from build123d import *

# Parameters (mm, degrees)
BOSS_EXTRUDE2_DEPTH = 50.25
CUT_EXTRUDE3_DEPTH  = 37
SKETCH6_W           = 6.4
SKETCH6_H           = 6.4
SKETCH6_R           = 1.7
BOSS_EXTRUDE3_DEPTH = 3
SKETCH8_W           = 102.5
SKETCH8_H           = 6.25
BOSS_EXTRUDE4_DEPTH = 2
SKETCH7_R           = 2
CUT_EXTRUDE4_DEPTH  = 7


with BuildPart() as part:
    # Sketch4 → Boss-Extrude2 (new body)
    with BuildSketch(Plane.XY):
        Polygon((3.25, 0), (105.75, 0), (105.75, 6.25), (103.25, 6.25), (103.25, 8.75), (109, 8.75), (109, 40), (0, 40), (0, 8.75), (5.75, 8.75), (5.75, 6.25), (3.25, 6.25), align=None)
    extrude(amount=BOSS_EXTRUDE2_DEPTH)

    # Sketch5 → Cut-Extrude3 (cut)
    with BuildSketch(Plane.XZ):
        Polygon((3.25, 0), (8.418575633, 0), (100.815935432, 0), (105.75, 0), (105.75, 45.25), (100.75, 45.25), (100.75, 47.25), (8.25, 47.25), (8.25, 45.25), (3.25, 45.25), align=None)
    extrude(amount=-CUT_EXTRUDE3_DEPTH, mode=Mode.SUBTRACT)

    # Sketch6 → Boss-Extrude3 (add)
    # profile 1 of 2: a face of its own
    with BuildSketch(Plane(origin=(0, 0, 0), x_dir=(-1, 0, 0), z_dir=(0, 0, -1))):
        with Locations((-105.8, 43.2)):
            Rectangle(SKETCH6_W, SKETCH6_H)
        with Locations((-105.8, 43.2)):
            Circle(SKETCH6_R, mode=Mode.SUBTRACT)
    # profile 2 of 2: a face of its own
    with BuildSketch(Plane(origin=(0, 0, 0), x_dir=(-1, 0, 0), z_dir=(0, 0, -1))):
        with Locations((-3.2, 43.2)):
            Rectangle(SKETCH6_W, SKETCH6_H)
        with Locations((-3.2, 43.2)):
            Circle(SKETCH6_R, mode=Mode.SUBTRACT)
    extrude(amount=-BOSS_EXTRUDE3_DEPTH)

    # Sketch8 → Boss-Extrude4 (add)
    with BuildSketch(Plane.XY.offset(50.25)):
        with Locations((54.5, 3.125)):
            Rectangle(SKETCH8_W, SKETCH8_H)
    extrude(amount=BOSS_EXTRUDE4_DEPTH)

    # Sketch7 → Cut-Extrude4 (cut)
    with BuildSketch(Plane(origin=(105.75, 0, 0), x_dir=(0, 0, -1), z_dir=(1, 0, 0))):
        with Locations((-48.75, 3.125)):
            Circle(SKETCH7_R)
    cut_extrude4 = extrude(amount=-CUT_EXTRUDE4_DEPTH, mode=Mode.SUBTRACT)

    # Mirror1: Cut-Extrude4 across plane
    add(cut_extrude4.mirror(Plane(origin=(54.5, 0, 0), x_dir=(0, 0, 1), z_dir=(1, 0, 0))), mode=Mode.SUBTRACT)


solid = part.part
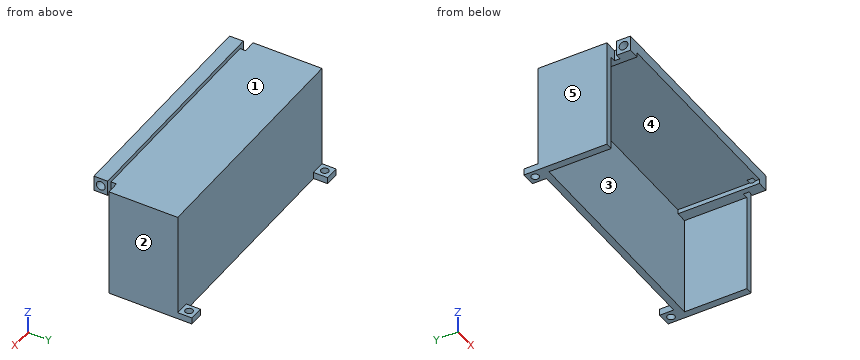
Source: CAD feature listing. Evaluate the final solid. Frame: model axes, mm. Face numbers are marked on the shaded views. A direction names the side the tool comes from. Round coordinates to 2 decimals unless told otherwise and drop trailing zeros. Order: outer loops, then holes, each group sorted by start corner. A loop starts at its lowest first (then second) coordinate and runs counter-clockwise, first axis right, second up. Notation, with made-up numbers: (-37.5, -16.5) - (-28.5, -16.5) arc R15 cw to (-28.5, -1.5) - close; hole circle Ø6 at (49.25, 43). An arc over 180 degrees is marked (long way). Use a Markdown table: item, result. Add a question column.
1. Section query A-A (y = 43.2). Return the cut outline in (x, z).
2. Set-up query: the marked faces 4 and 5. Return all of +Z, -Z, +X, -X, +Y, -Y with unobstructed straight access to the full face (end or side cutting, diameter ignored); none if empty.
3. Mould query, pull axis X, two halves, no side actions, for the marked faces 1, 2 and 3. Classes: +X half, -X half, draft (parallel to the pull), parting line (faces both ways), or undercut.
4. First-contact query: pin 1 (1.9 mm diameter, centred on y = 4, z = 49, fed in from -X); pin 2 (6.5 mm diameter, centred on y = 3.125, z = 48.75, fed in from +X); pin 3 (1 mm diameter, centred on x = 82.5, y = 33, fed in from +Z). Flat tips, straight axial feed; report the tip coordinate or a pass-through.
5. Section query C-C (z = 48.75). Return the cut outline in (x, y) (3 decimals).
6. Section query D-D (y = 13.5). Return the cut outline in (x, z).
7. Section query B-B (x = 72). Return the cut outline in (y, z).
8. Line query: probe 1 along X at (y, z) = (43, 2); probe 2 along X at (y, z) = (26, 17.5); probe 3 along Y at (x, z) = (3.2, 1.8). Output: solid intervals per line, ascending.
Derived:
| question | item | result |
|---|---|---|
| 1 | outline | (0, 0) - (1.5, 0) - (1.5, 3) - (0, 3) - close; (4.9, 0) - (6.4, 0) - (6.4, 3) - (4.9, 3) - close; (102.6, 0) - (104.1, 0) - (104.1, 3) - (102.6, 3) - close; (107.5, 0) - (109, 0) - (109, 3) - (107.5, 3) - close |
| 2 | face 4 | -Z, -Y |
| 2 | face 5 | +Z, -Z, -X, +Y, -Y |
| 3 | face 1 | draft |
| 3 | face 2 | +X half |
| 3 | face 3 | undercut |
| 4 | pin 1 | x = 10.25 |
| 4 | pin 2 | x = 105.75 |
| 4 | pin 3 | z = 50.25 |
| 5 | outline | (0, 8.75) - (5.75, 8.75) - (5.75, 6.25) - (3.25, 6.25) - (3.25, 5.125) - (10.25, 5.125) - (10.25, 1.125) - (3.25, 1.125) - (3.25, 0) - (105.75, 0) - (105.75, 1.125) - (98.75, 1.125) - (98.75, 5.125) - (105.75, 5.125) - (105.75, 6.25) - (103.25, 6.25) - (103.25, 8.75) - (109, 8.75) - (109, 40) - (0, 40) - close |
| 6 | outline | (0, 0) - (3.25, 0) - (3.25, 45.25) - (8.25, 45.25) - (8.25, 47.25) - (100.75, 47.25) - (100.75, 45.25) - (105.75, 45.25) - (105.75, 0) - (109, 0) - (109, 50.25) - (0, 50.25) - close |
| 7 | outline | (0, 47.25) - (37, 47.25) - (37, 0) - (40, 0) - (40, 50.25) - (6.25, 50.25) - (6.25, 52.25) - (0, 52.25) - close |
| 8 | probe 1 | 0 to 1.51, 4.89 to 6.4, 102.6 to 104.11, 107.49 to 109 |
| 8 | probe 2 | 0 to 3.25, 105.75 to 109 |
| 8 | probe 3 | 8.75 to 41.5, 44.9 to 46.4 |
